Geometry: see drawing. Coordinates: mm, zero at the bounding-box minimum. Coordinates: 2 decimals unless noted, no trailing zeros. Write each loop counter-clockwise with the first axis right and the second up, starting at its lowest first coordinate (ties: lowest second). Pieces come first, ordered by that corner, then holes. Notation, with made-up numbers: (-12.75, 34.5) - (-3.75, 34.5) arc R14 cw to (-3.75, 57.5) - close; hole circle Ø7 at (22, 25). An arc over 180 degrees is marked (long way). Use a Markdown table: item, result. Add a question column.
Q1. Material intervals for probe 1 along X at (y, z) = (15.5, 2.05); probe 2 along Y at (x, z) = (25, 0.6) (1 decimal); probe 3 along Y at (x, z) = (3.75, 3.3), sorted ascending. Write a range as from..to.
Q2. Mould query, pull axis X, two halves, no side actions, for the marked faces 1, 2 and 3. Classes: released by +X, released by -X, zero draft, split by the parting line, or undercut.
Q3. Section query C-C (y = 15.5). Give the number of separate pieces and of enclosed holes in the cut face.
Q4. Section query B-B (z = 2.3). Return the cut outline in (x, y), then the cut area to 3 significant figures.
Q5. Section query D-D (x = 11). Return the cut outline in (y, z).
Q6. Section query A-A (z = 0.7). Return the cut outline in (x, y).
Q7. Pin query (flat end, axial travel): P1, Ø1.5, axis at x = 19.5, z = 1, coming from the +Y side; P2, Ø1, axis at x = 3.5, y = 6.5, coming from the -Z side. Return the tip coordinate at first contact, or that it passes through.
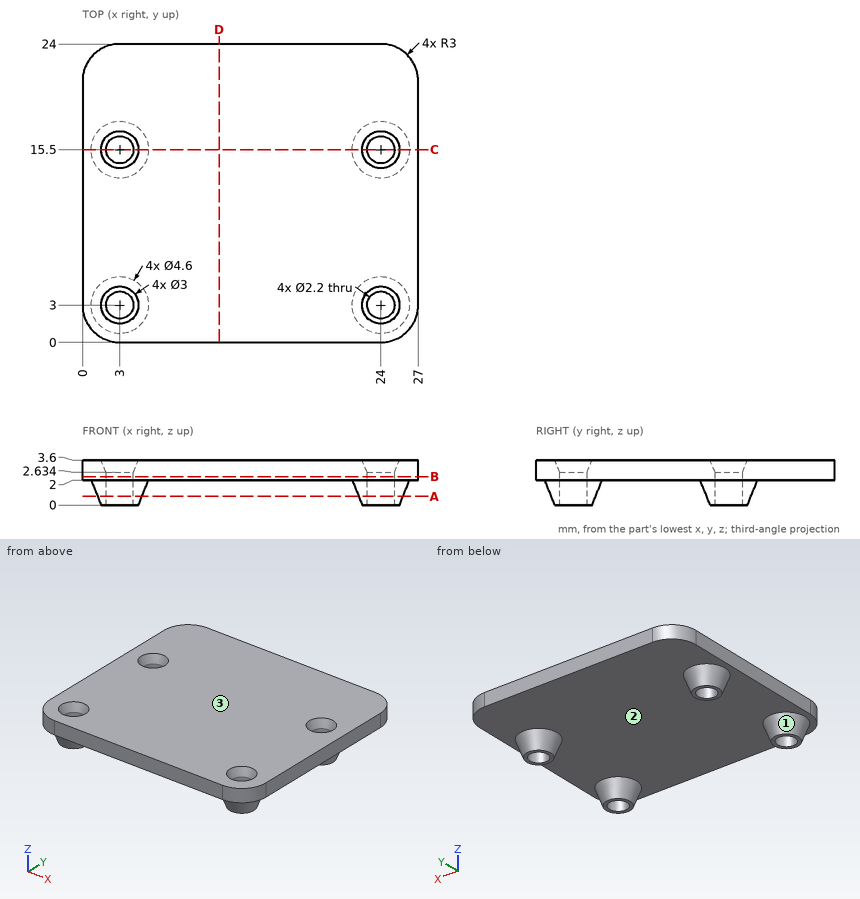
Values follow:
| question | item | result |
|---|---|---|
| 1 | probe 1 | 0..1.9, 4.1..22.9, 25.1..27 |
| 1 | probe 2 | 1.6..2.5, 3.5..4.4, 14.1..15, 16..16.9 |
| 1 | probe 3 | 0..1.85, 4.15..14.35, 16.65..24 |
| 2 | face 1 | undercut |
| 2 | face 2 | undercut |
| 2 | face 3 | zero draft |
| 3 | separate pieces | 3 |
| 3 | enclosed holes | 0 |
| 4 | outline | (0, 3) arc R3 ccw to (3, 0) - (24, 0) arc R3 ccw to (27, 3) - (27, 21) arc R3 ccw to (24, 24) - (3, 24) arc R3 ccw to (0, 21) - close; hole circle Ø2.2 at (3, 3); hole circle Ø2.2 at (3, 15.5); hole circle Ø2.2 at (24, 3); hole circle Ø2.2 at (24, 15.5) |
| 4 | area | 625 mm2 |
| 5 | outline | (0, 2) - (24, 2) - (24, 3.6) - (0, 3.6) - close |
| 6 | outline | circle Ø3.56 at (3, 3); circle Ø3.56 at (3, 15.5); circle Ø3.56 at (24, 3); circle Ø3.56 at (24, 15.5); hole circle Ø2.2 at (3, 3); hole circle Ø2.2 at (3, 15.5); hole circle Ø2.2 at (24, 3); hole circle Ø2.2 at (24, 15.5) |
| 7 | P1 | through |
| 7 | P2 | z = 2 |
